Verification items for the finished model (mm, model axes). A direction names the side the tool comes from. Round coordinates to 2 decimals unless told otherwise and drop trailing zeros. Order: outer loops, then holes, each group sorted by start corner. A loop starts at its lowest first (then second) coordinate and runs counter-clockwise, first axis right, second up. Notation, with made-up numbers: (12.5, -18) -> (32.5, -18) arc R23 cw to (32.5, 14) -> close; hole circle Ø4 at (82, 28). An arc over 180 degrees is marked (long way). Put each result on its own line as item: value.
from build123d import *

# Parameters (mm, degrees)
SKETCH1_W           = 75
SKETCH1_H           = 59
BOSS_EXTRUDE1_DEPTH = 2.032
SKETCH2_R           = 1.399999994
SKETCH2_R_2         = 1.4
BOSS_EXTRUDE2_DEPTH = 15


with BuildPart() as part:
    # Sketch1 → Boss-Extrude1 (new body)
    with BuildSketch(Plane(origin=(0, 0, 0), x_dir=(1, 0, 0), z_dir=(0, 1, 0))):
        with Locations((37.5, 29.5)):
            Rectangle(SKETCH1_W, SKETCH1_H)
    extrude(amount=-BOSS_EXTRUDE1_DEPTH)

    # Sketch2 → Boss-Extrude2 (add)
    with BuildSketch(Plane(origin=(0, 0, 0), x_dir=(1, 0, 0), z_dir=(0, 1, 0))):
        with Locations((2.5, 2.5)):
            Circle(SKETCH2_R)
        with Locations((72.5, 2.5)):
            Circle(SKETCH2_R_2)
        with Locations((72.5, 56.5)):
            Circle(SKETCH2_R_2)
        with Locations((2.5, 56.5)):
            Circle(SKETCH2_R)
    extrude(amount=BOSS_EXTRUDE2_DEPTH)


solid = part.part
Item 1: Section check B-B on x = 72.5. Record the boundary of the cut face in (y, z), then the cut area to 3 significant figures.
Check sheet entries:
outline: (-2.03, -59) -> (0, -59) -> (0, -57.9) -> (15, -57.9) -> (15, -55.1) -> (0, -55.1) -> (0, -3.9) -> (15, -3.9) -> (15, -1.1) -> (0, -1.1) -> (0, 0) -> (-2.03, 0) -> close
area: 204 mm^2
Item 2: Gauge pin test, flat ends, axial feed: pin 1 Ø10 at (x, y) = (57.5, 8.5) entering from -Z; pin 2 Ø17.5 at (x, z) = (38, -40.5) entering from +Y. Record the tip position at first contact, or that the pin passes through.
Check sheet entries:
pin 1: passes through
pin 2: stops at y = 0
Item 3: Section check A-A on z = -56.5. Record the boundary of the cut face in (x, y).
Check sheet entries:
outline: (0, -2.03) -> (75, -2.03) -> (75, 0) -> (73.9, 0) -> (73.9, 15) -> (71.1, 15) -> (71.1, 0) -> (3.9, 0) -> (3.9, 15) -> (1.1, 15) -> (1.1, 0) -> (0, 0) -> close
Item 4: Tool access check on faces 1 (the cylindrical face through (2.197, 7.395, -55.133)), 2 (the flat face through (72, 15, -3)). Record the directions out of +Z, -Z, +X, -X, +Y, -Y that give a thin tool (end or side, any length) a straight path to the whole face; none if there is none.
Check sheet entries:
face 1: +Y
face 2: +Z, -Z, +X, -X, +Y
Item 5: Section check C-C on y = 6.75. Record the boundary of the cut face in (x, z), then the cut area to 3 significant figures.
Check sheet entries:
outline: circle Ø2.8 at (2.5, -56.5); circle Ø2.8 at (2.5, -2.5); circle Ø2.8 at (72.5, -56.5); circle Ø2.8 at (72.5, -2.5)
area: 24.6 mm^2
Item 6: Material ranges on L1, parallel to Y at x = 11, z = -35.5, recorded low to high. Write a range as [from, to].
Check sheet entries:
L1: y = [-2.03, 0]
Item 7: Section check D-D on x = 44.5. Record the boundary of the cut face in (y, z), then the cut area to 3 significant figures.
Check sheet entries:
outline: (-2.03, -59) -> (0, -59) -> (0, 0) -> (-2.03, 0) -> close
area: 120 mm^2
Item 8: Release check for a two-part mould opening along X. For faces 3 (the cylindrical face through (3.25, 7.4, -3.68)), 4 (the flat face through (2, 15, -57)), 5 (the flat face through (0, -1, -29)) record: +X half, -X half, draft (parallel to the pull), parting line (faces both ways), or undercut.
Check sheet entries:
face 3: undercut
face 4: draft
face 5: -X half
